Geometry: final body of the model. Coordinates: model frame, mm. A direction names the side the tool comes from. Coordinates: 2 decimals unless noted, no trailing zeros. Order: outer loops, then holes, each group sorted by start corner. A loop starts at its lowest first (then second) coordinate and runs counter-clockwise, first axis right, second up. Notation, with made-up numbers: M 85,37 L 95,37 A15 cw 95,59 Z; hole C -35,56.25 d1. An arc over 180 degrees is marked long. Use CSV: the item, a comma, the result in double quotes. Start each with the question number.
Q1. First-contact query: P1, Ø2, axis at x = 45, y = -2.5, coming from the +Z side; P2, Ø2.5, axis at x = 4, z = 0, coming from the -Y side; P3, Ø2, axis at x = 21, z = 4.5, coming from the -Y side. Flat tips, straight axial feed; report the tip coordinate or a pass-through.
Q2. Access query for faces 1 (the face through (0, 0, 0)), 2 (the face through (50, 4, 4)). Directions: +Z, -Z, +X, -X, +Y, -Y. A direction counts if a zero-diameter tool reaches every point of the face in a straight line with its end or side. Return the directions, or none.
Q3. Ray query, probe 1 along X at (y, z) = (-3.4, 0); probe 2 along X at (y, z) = (-5.75, 2); probe 3 along X at (y, z) = (2.5, 0.75). Return the intervals inside material, ascending.
Q4. Section query B-B, the plane y = -4.75. Output: boundary loops of the cut face in (x, z).
Q5. Section query C-C, the plane x = 7. Output: boundary loops of the cut face in (y, z).
Q6. Section query A-A, the plane z = 0. Output: boundary loops of the cut face in (x, y).
Q7. Section query D-D, the plane z = -3.25. Output: boundary loops of the cut face in (x, y).
from build123d import *

# Parameters (mm, degrees)
SKETCH1_R               = 5.5
BOSS_EXTRUDE1_DEPTH     = 50
SKETCH2_R               = 7.5
BOSS_EXTRUDE2_DEPTH     = 5
SKETCH3_R               = 1
CUT_EXTRUDE1_DEPTH      = 8.5
CUT_EXTRUDE1_DEPTH_BACK = 8.5


with BuildPart() as part:
    # Sketch1 → Boss-Extrude1 (new body)
    with BuildSketch(Plane(origin=(0, 0, 0), x_dir=(0, 0, -1), z_dir=(1, 0, 0))):
        Circle(SKETCH1_R)
    extrude(amount=BOSS_EXTRUDE1_DEPTH)

    # Sketch2 → Boss-Extrude2 (add)
    with BuildSketch(Plane(origin=(50, 0, 0), x_dir=(0, 0, -1), z_dir=(1, 0, 0))):
        Circle(SKETCH2_R)
    extrude(amount=BOSS_EXTRUDE2_DEPTH)

    # Sketch3 → Cut-Extrude1 (cut, two sides)
    with BuildSketch(Plane(origin=(0, 0, 0), x_dir=(1, 0, 0), z_dir=(0, 1, 0))) as cut_extrude1_sk:
        with Locations((4, 0)):
            Circle(SKETCH3_R)
    extrude(amount=CUT_EXTRUDE1_DEPTH, mode=Mode.SUBTRACT)
    extrude(cut_extrude1_sk.sketch, amount=-CUT_EXTRUDE1_DEPTH_BACK, mode=Mode.SUBTRACT)


solid = part.part
Responses:
1,P1,"stops at z = 5.29"
1,P2,"stops at y = -5.5"
1,P3,"stops at y = -4.24"
2,face 1,"+Z, -Z, -X, +Y, -Y"
2,face 2,"-X"
3,probe 1,"x = 0 to 3, 5 to 55"
3,probe 2,"x = 50 to 55"
3,probe 3,"x = 0 to 3.34, 4.66 to 55"
4,outline,"M 0,-2.77 L 50,-2.77 L 50,-5.8 L 55,-5.8 L 55,5.8 L 50,5.8 L 50,2.77 L 0,2.77 Z; hole C 4,0 d2"
5,outline,"C 0,0 d11"
6,outline,"M 0,-5.5 L 3,-5.5 L 3,5.5 L 0,5.5 Z; M 5,-5.5 L 50,-5.5 L 50,-7.5 L 55,-7.5 L 55,7.5 L 50,7.5 L 50,5.5 L 5,5.5 Z"
7,outline,"M 0,-4.44 L 50,-4.44 L 50,-6.76 L 55,-6.76 L 55,6.76 L 50,6.76 L 50,4.44 L 0,4.44 Z"
